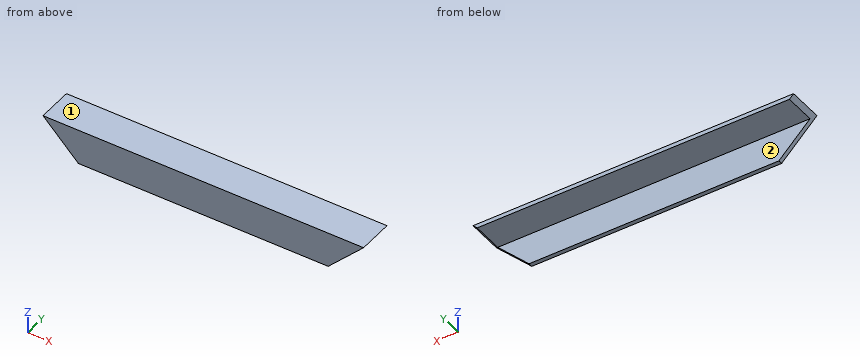
from build123d import *

# Parameters (mm, degrees)
SALIENTE_EXTRUIR1_DEPTH = 230
CORTAR_EXTRUIR1_DEPTH   = 75


with BuildPart() as part:
    # Croquis1 → Saliente-Extruir1 (new body)
    with BuildSketch(Plane(origin=(0, 0, 0), x_dir=(0, 0, -1), z_dir=(1, 0, 0))):
        Polygon((-16.874298957, 6.35), (-16.874298957, -19.05), (8.525701043, -19.05), (8.525701043, -16.05), (-13.874298957, -16.05), (-13.874298957, 6.35), align=None)
    extrude(amount=SALIENTE_EXTRUIR1_DEPTH)

    # Croquis2 → Cortar-Extruir1 (cut)
    with BuildSketch(Plane(origin=(0, 6.35, 0), x_dir=(1, 0, 0), z_dir=(0, 1, 0))):
        Polygon((0, -16.874298957), (25.4, 8.525701043), (0, 8.525701043), align=None)
        Polygon((230, -16.874298957), (204.6, 8.525701043), (230, 8.525701043), align=None)
    extrude(amount=-CORTAR_EXTRUIR1_DEPTH, mode=Mode.SUBTRACT)


solid = part.part
Design review of the part built by this model. Coordinates are the model's own, in mm. Face numbers are marked on the shaded views. A direction names the side the tool comes from. Round coordinates to 2 decimals unless told otherwise and drop trailing zeros. Write each loop counter-clockwise with the first axis right and the second up, starting at its lowest first coordinate (ties: lowest second). Pieces come first, ordered by that corner, then holes. Notation, with made-up numbers: (50, 80) - (73, 80) arc R22 ccw to (73, 103) - close; hole circle Ø2 at (-23, -28). An arc over 180 degrees is marked (long way). Use a Markdown table: item, result. Add a question column.
1. We need section C-C (z = -5.25). State the section outline as (x, y) points, then the cut area to 3 significant figures.
2. For the marked faces 1 and 2, list the 3-axis set-ups (+Z, -Z, +X, -X, +Y, -Y) from which the entire face can be reached by the end or side of a thin tool; tool diameter is ignored.
3. Clearance check with flat-ended pins moving along their axes: pin 1 (1 mm diameter, centred on y = -7.5, z = 12.5, fed in from +X); pin 2 (6.5 mm diameter, centred on x = 144, z = 4.5, fed in from +Y); pin 3 (1 mm diameter, centred on y = -16.5, z = -4, fed in from +X); pin 4 (6 mm diameter, centred on x = 164, z = 11, fed in from +Y). State where each tip first meets the part, or that it passes through.
4. We need section A-A (x = 117). State the section outline as (y, z) points, then the cut area to 3 significant figures.
5. Wall thickness on probe 1 along Y at (x, z) = (55.5, -3); probe 2 along Z at (x, y) = (217.5, -4); probe 3 along X at (y, z) = (-17.75, 10.25): over which ranges is each line inside the solid? List them lowest first.
6. We need section B-B (y = -5). State the section outline as (x, z) points.
Output:
| question | item | result |
|---|---|---|
| 1 | outline | (22.12, -19.05) - (207.88, -19.05) - (207.88, -16.05) - (22.12, -16.05) - close |
| 1 | area | 557 mm2 |
| 2 | face 1 | +Z, +X, -X, +Y, -Y |
| 2 | face 2 | -Z, +X, -X, +Y |
| 3 | pin 1 | passes through |
| 3 | pin 2 | stops at y = -16.05 |
| 3 | pin 3 | stops at x = 209.63 |
| 3 | pin 4 | stops at y = 6.35 |
| 4 | outline | (-19.05, -8.53) - (-16.05, -8.53) - (-16.05, 13.87) - (6.35, 13.87) - (6.35, 16.87) - (-19.05, 16.87) - close |
| 4 | area | 143 mm2 |
| 5 | probe 1 | y = -19.05 to -16.05 |
| 5 | probe 2 | z = 13.87 to 16.87 |
| 5 | probe 3 | x = 6.62 to 223.38 |
| 6 | outline | (0, 16.87) - (3, 13.87) - (227, 13.87) - (230, 16.87) - close |
